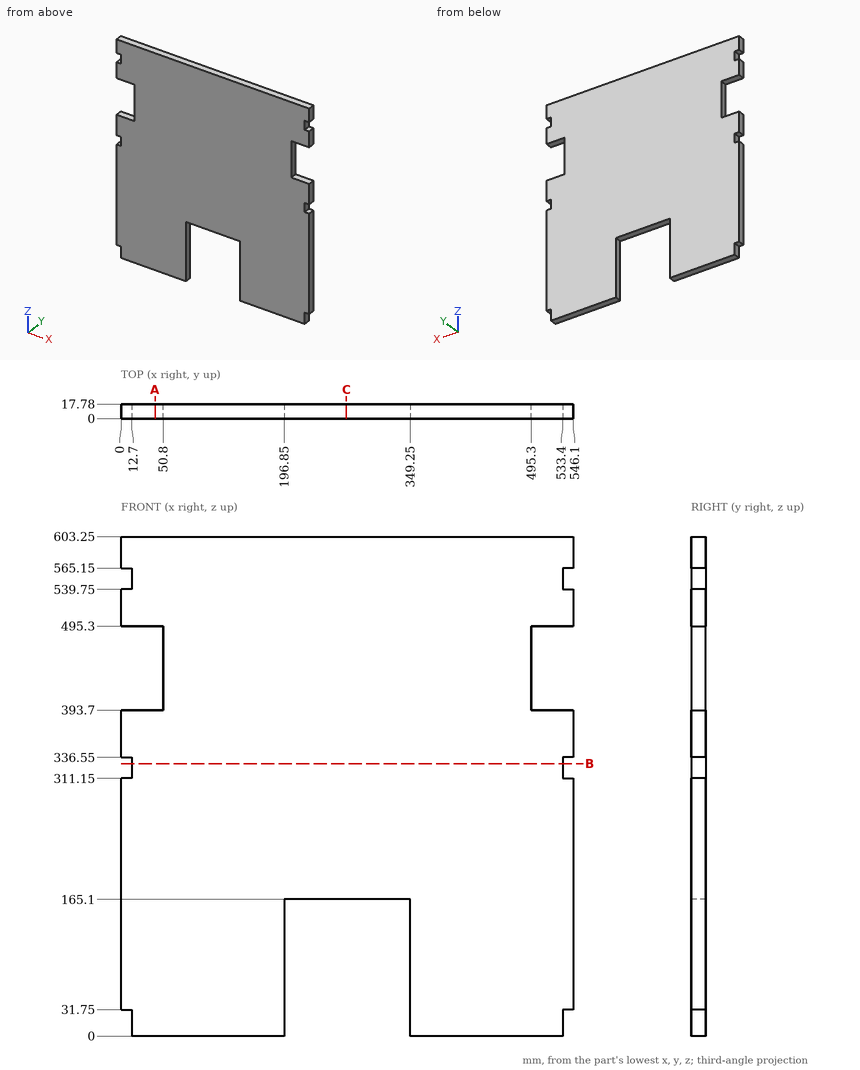
Job drawing, mm, ordinate dimensions from the low corner. One solid piece. Coordinates: 2 decimals unless noted, no trailing zeros. Order: outer loops, then holes, each group sorted by start corner. A loop starts at its lowest first (then second) coordinate and runs counter-clockwise, first axis right, second up. Notation, with made-up numbers: (21.25, 28) -> (56.25, 28) arc R7 ccw to (56.25, 35) -> close; hole circle Ø6 at (1, -32.75). An arc over 180 degrees is marked (long way). Answer in a Markdown table with one row per item. Add a question column.
Q1. Drop flat-ended pins along their axis: pin 1 (4 mm diameter, centred on x = 538.5, y = 11, fed in from -Z); pin 2 (5 mm diameter, centred on y = 4.5, z = 465, fed in from +X); pin 3 (9 mm diameter, centred on x = 275.5, y = 12, fed in from -Z). Give the stop position or say it passes through.
Q2. Band-saw the part on A-A, the plane x = 41. List the corners of the cut face in (y, z), then the cut area to 3 significant figures.
Q3. Band-saw the part on C-C, the plane x = 272. List the corners of the cut face in (y, z), then the cut area to 3 significant figures.
Q4. Wall check: line 1 along X through (y, z) = (11.25, 103); line 2 along Z through (x, y) = (49, 7.5); line 3 along Z through (x, y) = (337.5, 8). Give the ranges that are in metal, low to high. Write a range as [from, to].
Q5. Band-saw the part on B-B, the plane z = 329. List the corners of the cut face in (x, y).
Answers follow:
| question | item | result |
|---|---|---|
| 1 | pin 1 | z = 31.75 |
| 1 | pin 2 | x = 495.3 |
| 1 | pin 3 | z = 165.1 |
| 2 | outline | (0, 0) -> (17.78, 0) -> (17.78, 393.7) -> (0, 393.7) -> close; (0, 495.3) -> (17.78, 495.3) -> (17.78, 603.25) -> (0, 603.25) -> close |
| 2 | area | 8,920 mm^2 |
| 3 | outline | (0, 165.1) -> (17.78, 165.1) -> (17.78, 603.25) -> (0, 603.25) -> close |
| 3 | area | 7,790 mm^2 |
| 4 | line 1 | [0, 196.85], [349.25, 546.1] |
| 4 | line 2 | [0, 393.7], [495.3, 603.25] |
| 4 | line 3 | [165.1, 603.25] |
| 5 | outline | (12.7, 0) -> (533.4, 0) -> (533.4, 17.78) -> (12.7, 17.78) -> close |
